Here's the drawing with two shaded views (mm, measured from the low corner). I have some questions. Coordinates: 2 decimals unless noted, no trailing zeros. Loops run counter-clockwise (first coordinate to the right, second up) from the corner with the lowest first, then second, coordinate; pieces in that order, holes last. Notation, with made-up numbers: (50, 82) - (73, 82) arc R19 ccw to (73, 90) - close; hole circle Ø11 at (17, 1.5). An arc over 180 degrees is marked (long way). One line per item, written item: value. Start each with the question number.
(1) I'm going to push a flat-ended pin straight in: P1, Ø1.5, axis at y = 6, z = 1, coming from the -X side. Where does the tip first touch, or does it pass through?
(2) If we section it at A-A on y = 48: Write out the boundary of the cut face in (x, z), then the cut area to 3 significant figures.
(3) If I drill on line 1 along Y through (x, z) = (4, 2.3); line 2 along X through (y, z) = (9, 0.2); line 3 along Y through (x, z) = (0.5, 2.6), over which ranges is the centre line in solid material (lowest first)? Write a range as from..to.
(4) If we section it at B-B on x = 4: Write out the boundary of the cut face in (y, z).
(5) If we section it at D-D on y = 11.5: Write out the boundary of the cut face in (x, z).
(6) If we section it at C-C on z = 0.95: Write out the boundary of the cut face in (x, y), then the cut area to 3 significant figures.
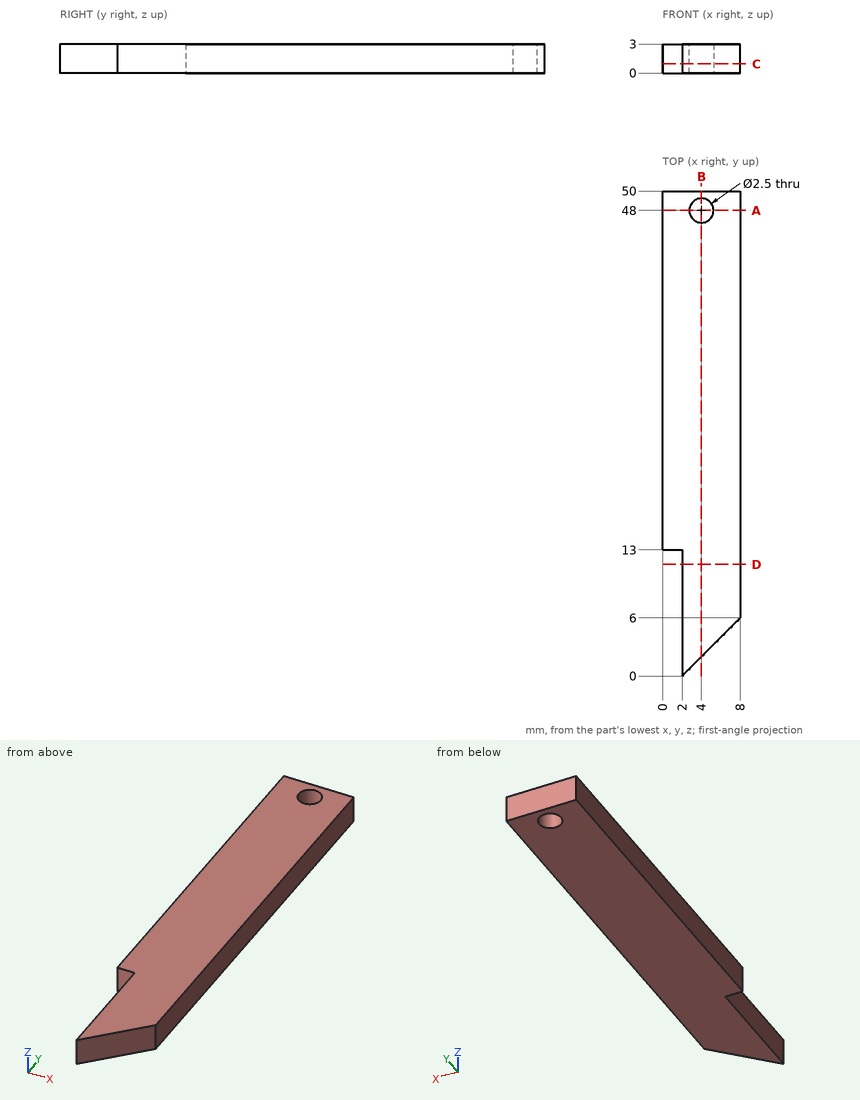
Values:
1. P1: stops at x = 2
2. outline: (0, 0) - (2.75, 0) - (2.75, 3) - (0, 3) - close; (5.25, 0) - (8, 0) - (8, 3) - (5.25, 3) - close
2. area: 16.5 mm2
3. line 1: y = 2..46.75, 49.25..50
3. line 2: x = 2..8
3. line 3: y = 13..50
4. outline: (2, 0) - (46.75, 0) - (46.75, 3) - (2, 3) - close; (49.25, 0) - (50, 0) - (50, 3) - (49.25, 3) - close
5. outline: (2, 0) - (8, 0) - (8, 3) - (2, 3) - close
6. outline: (0, 13) - (2, 13) - (2, 0) - (8, 6) - (8, 50) - (0, 50) - close; hole circle Ø2.5 at (4, 48)
6. area: 351 mm2
